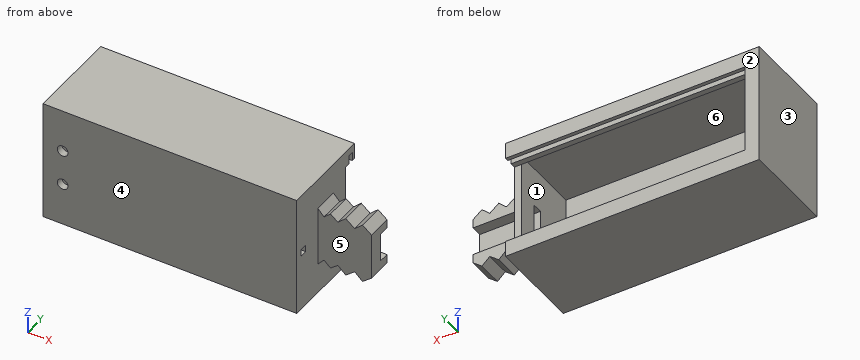
Autodesk Inventor part; units mm, degrees
ref_plane "工作平面1" through (0, 13, 0) normal (0, 1, 0) x (1, 0, 0)
ref_plane "YZ Plane" through (0, 0, 0) normal (1, 0, 0) x (0, 1, 0)
ref_plane "XZ Plane" through (0, 0, 0) normal (0, 1, 0) x (-1, 0, 0)
sketch "草图1" plane through (0, 0, 0) normal (0, 1, 0) x (-1, 0, 0)
  line L0 (0, 0) -> (0, -6.5)
  line L1 (0, 0) -> (15, 0)
  line L2 (0, 0) -> (0, -6.5)
  line L3 (0, -6.5) -> (2.5, -8.5)
  line L4 (2.5, -8.5) -> (4.6956, -6.5)
  line L5 (4.6956, -6.5) -> (7.1956, -8.5)
  line L6 (7.1956, -8.5) -> (9.3913, -6.5)
  line L7 (9.3913, -6.5) -> (11.4564, -8.1521)
  line L8 (11.4564, -8.1521) -> (13.2702, -6.5)
  line L9 (13.2702, -6.5) -> (15, -8.399)
  line L10 (15, 0) -> (82, 0)
  line L11 (82, 0) -> (82, -17)
  line L12 (82, -17) -> (15, -17)
  line L13 (15, -17) -> (15, -8.399)
  line L14 (15, -10) -> (15, -8.399)
  line L15 (15, -10) -> (15, -8.399)
  dimension "d1" = 6.5
  dimension "d2" = 15
  dimension "d3" = 99.01
  dimension "d4" = 67
  dimension "d6" = 17
extrude "拉伸1" add sketch "草图1" along normal blind 26
sketch "草图2" plane through (-82, 0, -17) normal (-1, 0, 0) x (0, 0, 1)
  line L0 (4.4791, 22) -> (2, 22)
  line L1 (2, 22) -> (2, 2)
  line L2 (2, 2) -> (17, 2)
  line L3 (4.4791, 23.5) -> (2, 23.5)
  line L4 (2, 23.5) -> (2, 25)
  line L5 (2, 25) -> (4.4791, 25)
  line L6 (0, 0) -> (17, 0)
  line L7 (17, 0) -> (17, 26)
  line L8 (0, 26) -> (17, 26)
  line L9 (0, 0) -> (0, 26)
  line L10 (4.4791, 25) -> (4.4791, 26)
  line L11 (4.4791, 23.5) -> (4.4791, 22)
  line L12 (17, 0) -> (17, 26)
  line L13 (4.4791, 26) -> (17, 26)
  line L14 (17, 26) -> (17, 2)
  dimension "d9" = 20
  dimension "d11" = 1.5
  dimension "d12" = 1.5
  dimension "d13" = 15
  dimension "d14" = 2
extrude "拉伸2" cut sketch "草图2" against normal blind 65 contours L11 L3 L4 L5 L10 L8 L7 L2 L1 L0
sketch "草图3" plane through (-82, 0, -17) normal (-1, 0, 0) x (0, 0, 1)
  line L0 (0, 0) -> (0, 26)
  line L1 (0, 26) -> (17, 26)
  line L2 (17, 26) -> (17, 0)
  line L3 (17, 0) -> (0, 0)
  line L4 (0, 0) -> (0, 26)
extrude "拉伸3" add sketch "草图3" along normal blind 4
mirror "镜像1" about plane through (-82, 0, 0) normal (0, 0, 1) of "拉伸1", "拉伸2", "拉伸3"
sketch "草图4" plane through (0, 26, 0) normal (0, 1, 0) x (1, 0, 0)
  line L0 (-15, -17) -> (-86, -17)
  line L1 (-15, -8.399) -> (-15, -17)
  line L2 (-13.2702, -6.5) -> (-15, -8.399)
  line L3 (-11.4564, -8.1521) -> (-13.2702, -6.5)
  line L4 (-9.3913, -6.5) -> (-11.4564, -8.1521)
  line L5 (-7.1956, -8.5) -> (-9.3913, -6.5)
  line L6 (-4.6956, -6.5) -> (-7.1956, -8.5)
  line L7 (-2.5, -8.5) -> (-4.6956, -6.5)
  line L8 (0, -6.5) -> (-2.5, -8.5)
  line L9 (0, 6.5) -> (0, -6.5)
  line L10 (0, 6.5) -> (-2.5, 8.5)
  line L11 (-2.5, 8.5) -> (-4.6956, 6.5)
  line L12 (-4.6956, 6.5) -> (-7.1956, 8.5)
  line L13 (-7.1956, 8.5) -> (-9.3913, 6.5)
  line L14 (-9.3913, 6.5) -> (-11.4564, 8.1521)
  line L15 (-11.4564, 8.1521) -> (-13.2702, 6.5)
  line L16 (-13.2702, 6.5) -> (-15, 8.399)
  line L17 (-15, 8.399) -> (-15, 17)
  line L18 (-15, 17) -> (-86, 17)
  line L19 (-86, 17) -> (-86, -17)
  line L20 (-82, 12.5209) -> (-82, -12.5209)
  line L21 (-82, 12.5209) -> (-17, 12.5209)
  line L22 (-17, 12.5209) -> (-17, -12.5209)
  line L23 (-17, -12.5209) -> (-82, -12.5209)
  line L24 (-15, -8.399) -> (-15, 8.399)
  point P0 (0, 0)
extrude "拉伸4" cut sketch "草图4" against normal blind 9.5 contours L24 L16 L15 L14 L13 L12 L11 L10 L9 L8 L7 L6 L5 L4 L3 L2
ref_plane "工作平面1" through (0, 13, 0) normal (0, 1, 0) x (1, 0, 0)
mirror "镜像2" about plane through (0, 13, 0) normal (0, 1, 0) of "拉伸4"
sketch "草图5" plane through (-15, 0, -17) normal (1, 0, 0) x (0, 0, -1)
  line L0 (-32, 23.5) -> (-32, 25)
  line L1 (-4.4791, 23.5) -> (-2, 23.5)
  line L2 (-32, 25) -> (-2, 25)
  line L3 (-2, 25) -> (-2, 23.5)
  line L4 (-2, 23.5) -> (-32, 23.5)
  line L5 (-32, 23.5) -> (-32, 25)
  line L6 (-29.5209, 25) -> (-29.5209, 26)
  line L7 (-4.4791, 25) -> (-4.4791, 26)
  line L8 (-29.5209, 25) -> (-4.4791, 25)
  line L9 (-4.4791, 25) -> (-4.4791, 26)
  line L10 (-4.4791, 26) -> (-29.5209, 26)
  line L11 (-29.5209, 26) -> (-29.5209, 25)
  line L12 (-32, 22) -> (-29.5209, 22)
  line L13 (-29.5209, 22) -> (-4.4791, 22)
  line L14 (-4.4791, 22) -> (-4.4791, 23.5)
  line L15 (-4.4791, 23.5) -> (-29.5209, 23.5)
  line L16 (-29.5209, 23.5) -> (-29.5209, 22)
  point P0 (-17, 0)
extrude "拉伸5" cut sketch "草图5" against normal up to surface (2 mm away) from surface at 0
sketch "草图6" plane through (0, 16.5, 6.5) normal (1, 0, 0) x (0, 0, -1)
  line L0 (0, -7) -> (13, -7)
  line L1 (13, -7) -> (13, 0)
  line L2 (13, 0) -> (0, 0)
  line L3 (0, -7) -> (0, 0)
  line L4 (0, -3) -> (13, -3)
  line L5 (2.5, 0) -> (10.5, 0)
  line L6 (10.5, 0) -> (10.5, -3)
  line L7 (10.5, -3) -> (2.5, -3)
  line L8 (2.5, -3) -> (2.5, 0)
  line L9 (0, -7) -> (0, 0)
  line L10 (6.5, -3) -> (6.5, 0)
  line L11 (13, 0) -> (0, 0)
  dimension "d23" = 8
  dimension "d24" = 3
extrude "拉伸6" cut sketch "草图6" against normal blind 68.25 contours L8 L2 L10 L4 | L4 L10 L2 L6
sketch "草图7" plane through (0, 0, 0) normal (0, -1, 0) x (1, 0, 0)
  line L0 (-82, 15) -> (-82, -15)
  line L1 (-82, -15) -> (-17, -15)
  line L2 (-82, 15) -> (-17, 15)
  circle A0 centre (-80.5, -5) radius 1.5
  circle A1 centre (-80.5, 5) radius 1.5
  line L3 (-103.2, 0) -> (17.2, 0)
  point P0 (0, 0)
  dimension "d27" = 3
  dimension "d28" = 3
  dimension "d29" = 10
  dimension "d30" = 1.5
extrude "拉伸7" cut sketch "草图7" against normal blind 9.25
sketch "草图8" plane through (-15, 0, -17) normal (1, 0, 0) x (0, 0, -1)
  line L0 (-17.9721, 4) -> (-15.9721, 4)
  line L1 (-15.9721, 4) -> (-15.9721, 2)
  line L2 (-15.9721, 2) -> (-17.9721, 2)
  line L3 (-17.9721, 2) -> (-17.9721, 4)
  line L4 (-16.9721, 7.1271) -> (-16.9721, -1.5009)
  line L5 (0, 0) -> (-34, 0)
  point P0 (-17, 0)
  dimension "d33" = 2
  dimension "d34" = 2
  dimension "d35" = 2
extrude "拉伸8" cut sketch "草图8" against normal blind 5
properties part number "装置容器" material "银"
Model file for the job. Use its own axes, mm. Face numbers are marked on the shaded views. A direction names the side the tool comes from. Coordinates: 2 decimals unless noted, no trailing zeros. Write each loop counter-clockwise with the first axis right and the second up, starting at its lowest first coordinate (ties: lowest second). Pieces come first, ordered by that corner, then holes. Notation, with made-up numbers: (54.5, -22) - (71.5, -22) arc R34 ccw to (71.5, 12) - close; hole circle Ø10 at (-20, 55). An arc over 180 degrees is marked (long way). Use a Markdown table: item, result. Add a question column.
Item 1: 3-axis set-ups, long thin cutter, end or side, ignore diameter. For the marked faces 4, 5 and 6: which of +Z, -Z, +X, -X, +Y, -Y reach the whole face in a straight line?
Item 2: Band-saw the part on B-B, the plane x = -80.5. Write the cut outline in (y, z).
Item 3: Drop flat-ended pins along their axis: pin 1 (1.2 mm diameter, centred on x = -57.5, z = -14.5, fed in from -Y); pin 2 (1 mm diameter, centred on x = -25.5, z = 5, fed in from +Y); pin 3 (6.5 mm diameter, centred on x = -7.5, z = -1, fed in from +Y); pin 4 (3.5 mm diameter, centred on x = -7, y = 15.5, fed in from -Z). Give the stop position or say it passes through.
Item 4: Band-saw the part on D-D, the plane z = -10. Write the cut outline in (x, y).
Item 5: Band-saw the part on C-C, the plane z = 14. Write the cut outline in (x, y).
Item 6: Drill centre lines: line 1 along Z through (x, y) = (-80.5, 1); line 2 along Y through (x, z) = (-32, -14); line 3 along X through (y, z) = (0.75, 5). Where is each one in solid material? Low to high.
Item 7: Band-saw the part on A-A, the plane y = 12.5. Write the cut outline in (x, z).
Item 8: Two-plate mould, pull along X, no slides. Class the marked faces 1, 2 and 3: pulls with the +X half, pulls with the -X half, needs draft (parallel to the pull), parting line crosses it, or undercut.
A:
| question | item | result |
|---|---|---|
| 1 | face 4 | +Z, -Z, +X, -X, -Y |
| 1 | face 5 | +Z, -Z, +X, -Y |
| 1 | face 6 | none |
| 2 | outline | (0, -17) - (26, -17) - (26, -12.52) - (25, -12.52) - (25, -15) - (23.5, -15) - (23.5, -12.52) - (22, -12.52) - (22, -15) - (2, -15) - (2, -6.5) - (0, -6.5) - close; (0, -3.5) - (2, -3.5) - (2, 3.5) - (0, 3.5) - close; (0, 6.5) - (2, 6.5) - (2, 15) - (22, 15) - (22, 12.52) - (23.5, 12.52) - (23.5, 15) - (25, 15) - (25, 12.52) - (26, 12.52) - (26, 17) - (0, 17) - close |
| 3 | pin 1 | stops at y = 0 |
| 3 | pin 2 | stops at y = 2 |
| 3 | pin 3 | stops at y = 16.5 |
| 3 | pin 4 | stops at z = -8.5 |
| 4 | outline | (-86, 0) - (-15, 0) - (-15, 22) - (-17, 22) - (-17, 2) - (-82, 2) - (-82, 26) - (-86, 26) - close |
| 5 | outline | (-86, 0) - (-15, 0) - (-15, 23.5) - (-82, 23.5) - (-82, 25) - (-15, 25) - (-15, 26) - (-86, 26) - close; hole (-82, 2) - (-17, 2) - (-17, 22) - (-82, 22) - close |
| 6 | line 1 | z = -17 to -6.5, -3.5 to 3.5, 6.5 to 17 |
| 6 | line 2 | y = 0 to 2, 22 to 23.5, 25 to 26 |
| 6 | line 3 | x = -86 to -82, -79 to -15 |
| 7 | outline | (-86, -17) - (-15, -17) - (-15, -8.4) - (-13.27, -6.5) - (-11.46, -8.15) - (-9.39, -6.5) - (-7.2, -8.5) - (-4.7, -6.5) - (-2.5, -8.5) - (0, -6.5) - (0, 6.5) - (-2.5, 8.5) - (-4.7, 6.5) - (-7.2, 8.5) - (-9.39, 6.5) - (-11.46, 8.15) - (-13.27, 6.5) - (-15, 8.4) - (-15, 17) - (-86, 17) - close; hole (-82, -15) - (-17, -15) - (-17, 15) - (-82, 15) - close |
| 8 | face 1 | undercut |
| 8 | face 2 | needs draft |
| 8 | face 3 | pulls with the -X half |
